Can you work these out from the model? Positions are in its coordinate system, mm. Face numbers are marked on the shaded views. A direction names the side the tool comes from. Round coordinates to 2 decimals unless told otherwise and drop trailing zeros. Write each loop counter-clockwise with the first axis right and the second up, starting at its lowest first coordinate (ties: lowest second). Pieces come first, ordered by that corner, then holes. Notation, with made-up numbers: M 5,9 L 11,9 A22 cw 11,15 Z; hole C -16,20.25 d10. An arc over 180 degrees is marked long. Answer as a JSON object with one key per item and string values. Group by question number.
1) Suppose I cut it at D-D, the plane x = 0. Write out the boundary of the cut face in (y, z).
2) Suppose I cut it at A-A, the plane x = -19. Write out the boundary of the cut face in (y, z).
3) I'm going to push flat-ended pins straight in: pin 1 Ø4 at (y, z) = (-8.5, 12) entering from -X; pin 2 Ø8 at (y, z) = (-5, 2) entering from +X; pin 3 Ø1 at (x, y) = (-11.5, -4) entering from +Z; pin 4 Ø2.5 at (x, y) = (-19, -9.5) entering from -Z. Where does each tip first touch, or does it pass through?
4) Suppose I cut it at B-B, the plane z = 5.25. Write out the boundary of the cut face in (x, y).
5) On a 3-axis mill with a long thin cutter (end or side, diameter ignored), from which of +Z, -Z, +X, -X, +Y, -Y can I reach the whole of each face in a straight line? I mean the marked faces 1, 2, 3 and 4. Say none if no direction works.
6) If we mould it in two halves opening along X, with no side actions, what happens to the marked faces 5, 6 and 7? For each: +X half, -X half, draft (parallel to the pull), parting line (faces both ways), or undercut.
7) Please list where these lines run through material, in increasing order: L1, parallel to X at y = -9.5, z = 0.25; L2, parallel to X at y = -11.5, z = 1.5; L3, parallel to Y at x = 19, z = 0.5. Write a range as [from, to].
8) Suppose I cut it at C-C, the plane y = -9. Write out the boundary of the cut face in (x, z), and give its area (3 significant figures).
from build123d import *

# Parameters (mm, degrees)
F1_DEPTH = 19
F2_R     = 2
F3_DEPTH = 25


with BuildPart() as f1:
    # F0 (on Front) → F1 (new body)
    with BuildSketch(Plane.XZ):
        with BuildLine():
            ThreePointArc((-7.5, 7.5), (0, 15), (7.5, 7.5))
            Line((7.5, 7.5), (7.5, 0))
            Line((7.5, 0), (24.5, 0))
            Line((24.5, 0), (24.5, 0.8))
            Line((24.5, 0.8), (12.25, 0.8))
            Line((12.25, 0.8), (12.25, 7.5))
            ThreePointArc((12.25, 7.5), (0, 19.75), (-12.25, 7.5))
            Line((-12.25, 7.5), (-12.25, 0.8))
            Line((-12.25, 0.8), (-24.5, 0.8))
            Line((-24.5, 0.8), (-24.5, 0))
            Line((-24.5, 0), (-7.5, 0))
            Line((-7.5, 0), (-7.5, 7.5))
        make_face()
    extrude(amount=F1_DEPTH)

    # F2 (on face) → F3 (cut)
    with BuildSketch(Plane(origin=(0, 0, 0), x_dir=(1, 0, 0), z_dir=(0, 0, -1))):
        with Locations((-19, 9.5)):
            Circle(F2_R)
        with Locations((19, 9.5)):
            Circle(F2_R)
        with BuildLine():
            ThreePointArc((-22.58318, 0), (-24.016014, 4.654275), (-24.5, 9.5))
            Line((-24.5, 9.5), (-24.5, 0))
            Line((-24.5, 0), (-22.58318, 0))
        make_face()
        with BuildLine():
            ThreePointArc((-24.5, 9.5), (-24.016014, 14.345725), (-22.58318, 19))
            Line((-22.58318, 19), (-24.5, 19))
            Line((-24.5, 19), (-24.5, 9.5))
        make_face()
        with BuildLine():
            ThreePointArc((22.58318, 19), (24.5, 9.5), (22.58318, 0))
            Line((22.58318, 0), (24.50018, 0))
            Line((24.50018, 0), (24.50018, 19))
            Line((24.50018, 19), (22.58318, 19))
        make_face()
    extrude(amount=-F3_DEPTH, mode=Mode.SUBTRACT)


solid = f1.part
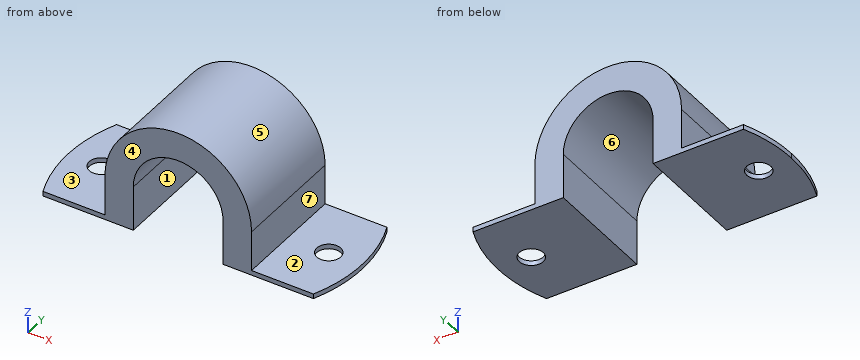
Results:
{
 "1": {"outline": "M -19,15 L 0,15 L 0,19.75 L -19,19.75 Z"},
 "2": {"outline": "M -19,0 L -11.5,0 L -11.5,0.8 L -19,0.8 Z; M -7.5,0 L 0,0 L 0,0.8 L -7.5,0.8 Z"},
 "3": {"pin 1": "x = -11.99", "pin 2": "x = 24.49", "pin 3": "z = 12.89", "pin 4": "through"},
 "4": {"outline": "M -12.25,-19 L -7.5,-19 L -7.5,0 L -12.25,0 Z; M 7.5,-19 L 12.25,-19 L 12.25,0 L 7.5,0 Z"},
 "5": {"face 1": "-Z, +Y, -Y", "face 2": "+Z, +X, +Y, -Y", "face 3": "+Z, -X, +Y, -Y", "face 4": "+Z, -Z, +X, -X, -Y"},
 "6": {"face 5": "parting line", "face 6": "undercut", "face 7": "+X half"},
 "7": {"L1": "[-24.5, -21], [-17, -7.5], [7.5, 17], [21, 24.5]", "L2": "[-12.25, -7.5], [7.5, 12.25]", "L3": "[-19, -11.5], [-7.5, 0]"},
 "8": {"outline": "M -24.49,0 L -20.94,0 L -20.94,0.8 L -24.49,0.8 Z; M -17.06,0 L -7.5,0 L -7.5,7.5 A7.5 cw 7.5,7.5 L 7.5,0 L 17.06,0 L 17.06,0.8 L 12.25,0.8 L 12.25,7.5 A12.25 ccw -12.25,7.5 L -12.25,0.8 L -17.06,0.8 Z; M 20.94,0 L 24.49,0 L 24.49,0.8 L 20.94,0.8 Z", "area": "232 mm^2"}
}
